Verification items for this drawing (mm, ordinates from the low corner). Round coordinates to 2 decimals unless told otherwise and drop trailing zeros. Write each loop counter-clockwise with the first axis right and the second up, starting at its lowest first coordinate (ties: lowest second). Pieces come first, ordered by that corner, then holes.
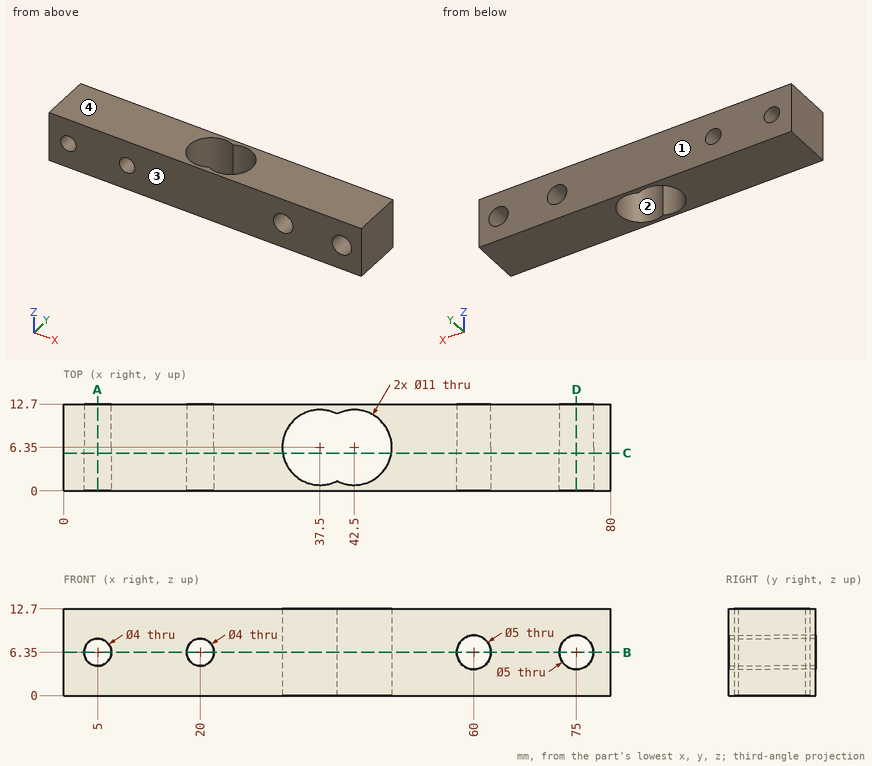
1. Release check for a two-part mould opening along Y. For the marked faces 1, 2, 3 and 4 record: +Y half, -Y half, draft (parallel to the pull), parting line (faces both ways), or undercut.
2. Section check D-D (x = 75). Record the cut outline in (y, z), plus the area to 3 significant figures.
3. Section check A-A (x = 5). Record the cut outline in (y, z).
4. Section check C-C (y = 5.5). Record the cut outline in (x, z), plus the area to 3 significant figures.
5. Section check B-B (z = 6.35). Record the cut outline in (x, y), plus the area to 3 significant figures.
6. Scan lines: line 1 along Z through (x, y) = (60, 5.25); line 2 along Y through (x, z) = (42.5, 6); line 3 along X through (y, z) = (3.5, 6.35). Record each from-to range of solid material in increasing order.
Results below:
1. face 1: +Y half
1. face 2: undercut
1. face 3: -Y half
1. face 4: draft
2. outline: (0, 0) - (12.7, 0) - (12.7, 3.85) - (0, 3.85) - close; (0, 8.85) - (12.7, 8.85) - (12.7, 12.7) - (0, 12.7) - close
2. area: 97.8 mm2
3. outline: (0, 0) - (12.7, 0) - (12.7, 4.35) - (0, 4.35) - close; (0, 8.35) - (12.7, 8.35) - (12.7, 12.7) - (0, 12.7) - close
4. outline: (0, 0) - (32.07, 0) - (32.07, 12.7) - (0, 12.7) - close; (47.93, 0) - (80, 0) - (80, 12.7) - (47.93, 12.7) - close; hole circle Ø4 at (5, 6.35); hole circle Ø4 at (20, 6.35); hole circle Ø5 at (60, 6.35); hole circle Ø5 at (75, 6.35)
4. area: 750 mm2
5. outline: (0, 0) - (3, 0) - (3, 12.7) - (0, 12.7) - close; (7, 0) - (18, 0) - (18, 12.7) - (7, 12.7) - close; (22, 0) - (57.5, 0) - (57.5, 12.7) - (22, 12.7) - close; (62.5, 0) - (72.5, 0) - (72.5, 12.7) - (62.5, 12.7) - close; (77.5, 0) - (80, 0) - (80, 12.7) - (77.5, 12.7) - close; hole (40, 1.45) arc R5.5 ccw (long way) to (40, 11.25) arc R5.5 ccw (long way) to start
5. area: 639 mm2
6. line 1: z = 0 to 3.85, 8.85 to 12.7
6. line 2: y = 0 to 0.85, 11.85 to 12.7
6. line 3: x = 0 to 3, 7 to 18, 22 to 32.8, 47.2 to 57.5, 62.5 to 72.5, 77.5 to 80
